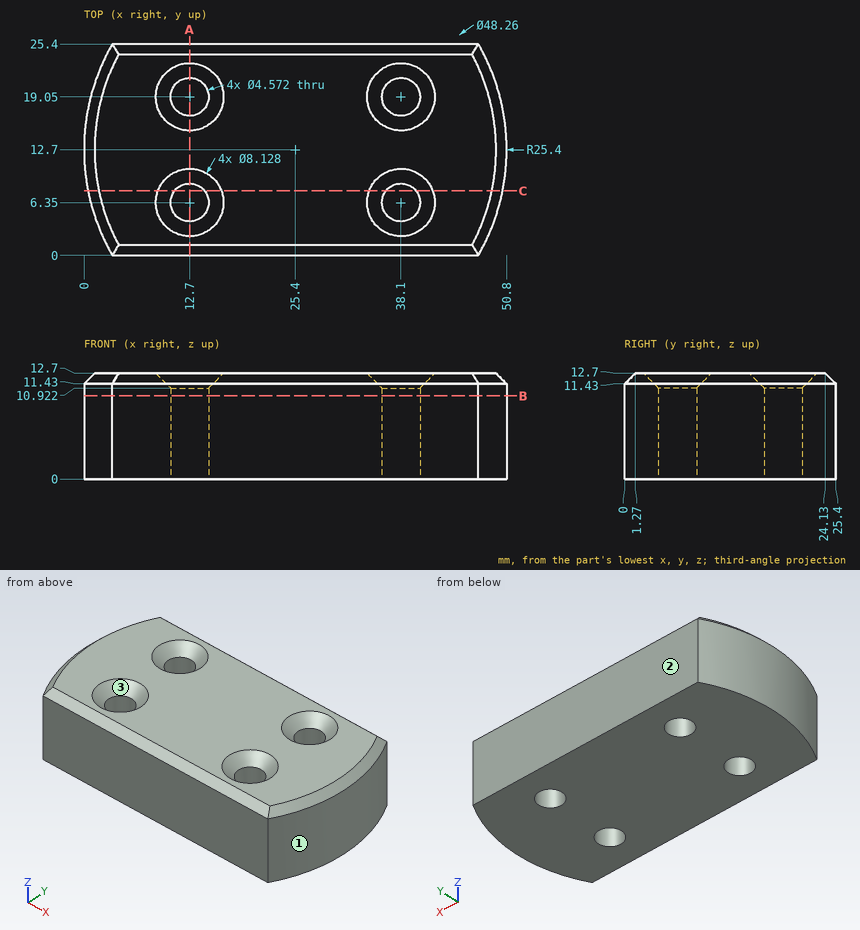
Here's the drawing with two shaded views (mm, measured from the low corner). I have some questions. Give positions to 0.01 mm unless a question says otherwise; leave off trailing zeros. Order: outer loops, then holes, each group sorted by start corner. A loop starts at its lowest first (then second) coordinate and runs counter-clockwise, first axis right, second up. Notation, with made-up numbers: (14, -14) -> (58, -14) arc R27 cw to (58, 14) -> close; hole circle Ø2 at (65, 84). An arc over 180 degrees is marked (long way). Use a Markdown table: item, result. Add a question column.
Item 1: I need wall thicknesses on line 1 (Y direction, x = 12.7, z = 2.5); line 2 (X direction, y = 20.5, z = 7.5); line 3 (X direction, y = 6.5, z = 5.5). Which ranges of each line are inside material? Lowest first, please.
Item 2: Will these pins go through, and if not, where does the flat tip stop? pin 1 (7.5 mm diameter, centred on x = 38.1, y = 6.35, fed in from +Z); pin 2 (5 mm diameter, centred on y = 4, z = 1.5, fed in from +X); pin 3 (4 mm diameter, centred on y = 20.5, z = 5.5, fed in from -X); pin 4 (12 mm diameter, centred on x = 13.5, y = 19.5, fed in from +Z).
Item 3: Imagine slicing it at C-C on y = 7.75. Give the number of separate pieces and of enclosed holes in the cut face, plus the area to 3 significant figures.
Item 4: If we mould it in two halves opening along Y, with no side actions, what happens to the marked faces 1, 2 and 3? For each: pulls with the +Y half, pulls with the -Y half, needs draft (parallel to the pull), parting line crosses it, or undercut.
Item 5: Imagine slicing it at B-B on z = 10. Please give me the cut outline in (x, y), plus the area to 3 significant figures.
Item 6: Imagine slicing it at A-A on x = 12.7. Please give me the cut outline in (y, z).
Data:
| question | item | result |
|---|---|---|
| 1 | line 1 | y = 0 to 4.06, 8.64 to 16.76, 21.34 to 25.4 |
| 1 | line 2 | x = 1.23 to 10.93, 14.47 to 36.33, 39.87 to 49.57 |
| 1 | line 3 | x = 0.77 to 10.42, 14.98 to 35.82, 40.38 to 50.03 |
| 2 | pin 1 | stops at z = 12.39 |
| 2 | pin 2 | stops at x = 50.03 |
| 2 | pin 3 | stops at x = 0.67 |
| 2 | pin 4 | stops at z = 12.7 |
| 3 | separate pieces | 3 |
| 3 | enclosed holes | 0 |
| 3 | area | 532 mm² |
| 4 | face 1 | parting line crosses it |
| 4 | face 2 | pulls with the +Y half |
| 4 | face 3 | undercut |
| 5 | outline | (3.4, 0) -> (47.4, 0) arc R25.4 ccw to (47.4, 25.4) -> (3.4, 25.4) arc R25.4 ccw to start; hole circle Ø4.57 at (12.7, 6.35); hole circle Ø4.57 at (12.7, 19.05); hole circle Ø4.57 at (38.1, 6.35); hole circle Ø4.57 at (38.1, 19.05) |
| 5 | area | 1,170 mm² |
| 6 | outline | (0, 0) -> (4.06, 0) -> (4.06, 10.92) -> (2.29, 12.7) -> (1.27, 12.7) -> (0, 11.43) -> close; (8.64, 0) -> (16.76, 0) -> (16.76, 10.92) -> (14.99, 12.7) -> (10.41, 12.7) -> (8.64, 10.92) -> close; (21.34, 0) -> (25.4, 0) -> (25.4, 11.43) -> (24.13, 12.7) -> (23.11, 12.7) -> (21.34, 10.92) -> close |
